Input: part model. Units: mm. Frame: model coordinates. Face numbers are marked on the shaded views. A direction names the side the tool comes from. Give positions to 0.01 mm unless a question says otherwise; leave off trailing zeros. Loops run counter-clockwise (first coordinate to the right, second up) from the corner with the lowest first, then second, coordinate; pieces in that order, holes last. Notation, with made-up numbers: (13, 3) -> (19, 3) arc R25 ccw to (19, 34) -> close; hole circle Ø11 at (-28, 33). An arc over 180 degrees is marked (long way). Answer as a JSON object with one key per item and string values.
Autodesk Fusion 360 part; units mm, degrees
sketch "Sketch1" plane through (0, 0, 0) normal (0, 0, 1) x (1, 0, 0)
  circle A0 centre (0, 0) radius 6.305 construction
  circle A1 centre (0, 0) radius 5.105 construction
  line L0 (0, 0) -> (0, 5.105) construction
  circle A2 centre (0, 5.995) radius 0.89 construction
  circle A3 centre (1.139, 5.9469) radius 0.25 construction
  line L1 (0, 0) -> (2.7356, 5.6806) construction
  line L2 (0, 0) -> (6.305, 0) construction
  circle A4 centre (2.6011, 5.4013) radius 0.89 construction
  circle A5 centre (1.5541, 5.8522) radius 0.25 construction
  arc A6 (0.9079, 5.9375) -> (0.8892, 5.9575) centre (0, 5.105) ccw construction
  arc A7 (0, 5.105) -> (0.8892, 5.9575) centre (0, 5.995) ccw
  arc A8 (1.186, 6.1924) -> (0.8892, 5.9575) centre (1.139, 5.9469) ccw
  arc A9 (1.7837, 5.7533) -> (1.6182, 6.0938) centre (1.5541, 5.8522) ccw
  arc A10 (1.7837, 5.7533) -> (2.215, 4.5994) centre (2.6011, 5.4013) ccw
  line L3 (1.186, 6.1924) -> (1.6182, 6.0938)
  arc A11 (-0.8892, 5.9575) -> (0, 5.105) centre (0, 5.995) ccw
  arc A12 (-0.8892, 5.9575) -> (-1.186, 6.1924) centre (-1.139, 5.9469) ccw
  line L4 (-1.6182, 6.0938) -> (-1.186, 6.1924)
  arc A13 (-1.6182, 6.0938) -> (-1.7837, 5.7533) centre (-1.5541, 5.8522) ccw
  arc A14 (-2.215, 4.5994) -> (-1.7837, 5.7533) centre (-2.6011, 5.4013) ccw
  arc A15 (-3.386, 4.9817) -> (-2.215, 4.5994) centre (-2.6011, 5.4013) ccw
  arc A16 (-3.386, 4.9817) -> (-3.7554, 5.0646) centre (-3.6065, 4.8638) ccw
  line L5 (-4.102, 4.7882) -> (-3.7554, 5.0646)
  arc A17 (-4.102, 4.7882) -> (-4.1033, 4.4096) centre (-3.9393, 4.5983) ccw
  arc A18 (-3.9912, 3.1829) -> (-4.1033, 4.4096) centre (-4.6871, 3.7378) ccw
  arc A19 (-5.2121, 3.0192) -> (-3.9912, 3.1829) centre (-4.6871, 3.7378) ccw
  arc A20 (-5.2121, 3.0192) -> (-5.5809, 2.9337) centre (-5.3596, 2.8173) ccw
  line L6 (-5.7733, 2.5342) -> (-5.5809, 2.9337)
  arc A21 (-5.7733, 2.5342) -> (-5.6102, 2.1926) centre (-5.5444, 2.4337) ccw
  arc A22 (-4.977, 1.136) -> (-5.6102, 2.1926) centre (-5.8447, 1.334) ccw
  arc A23 (-6.006, 0.4587) -> (-4.977, 1.136) centre (-5.8447, 1.334) ccw
  arc A24 (-6.006, 0.4587) -> (-6.3011, 0.2217) centre (-6.0513, 0.2129) ccw
  line L7 (-6.3011, -0.2217) -> (-6.3011, 0.2217)
  arc A25 (-6.3011, -0.2217) -> (-6.006, -0.4587) centre (-6.0513, -0.2129) ccw
  arc A26 (-4.977, -1.136) -> (-6.006, -0.4587) centre (-5.8447, -1.334) ccw
  arc A27 (-5.6102, -2.1926) -> (-4.977, -1.136) centre (-5.8447, -1.334) ccw
  arc A28 (-5.6102, -2.1926) -> (-5.7733, -2.5342) centre (-5.5444, -2.4337) ccw
  line L8 (-5.5809, -2.9337) -> (-5.7733, -2.5342)
  arc A29 (-5.5809, -2.9337) -> (-5.2121, -3.0192) centre (-5.3596, -2.8173) ccw
  arc A30 (-3.9912, -3.1829) -> (-5.2121, -3.0192) centre (-4.6871, -3.7378) ccw
  arc A31 (-4.1033, -4.4096) -> (-3.9912, -3.1829) centre (-4.6871, -3.7378) ccw
  arc A32 (-4.1033, -4.4096) -> (-4.102, -4.7882) centre (-3.9393, -4.5983) ccw
  line L9 (-3.7554, -5.0646) -> (-4.102, -4.7882)
  arc A33 (-3.7554, -5.0646) -> (-3.386, -4.9817) centre (-3.6065, -4.8638) ccw
  arc A34 (-2.215, -4.5994) -> (-3.386, -4.9817) centre (-2.6011, -5.4013) ccw
  arc A35 (-1.7837, -5.7533) -> (-2.215, -4.5994) centre (-2.6011, -5.4013) ccw
  arc A36 (-1.7837, -5.7533) -> (-1.6182, -6.0938) centre (-1.5541, -5.8522) ccw
  line L10 (-1.186, -6.1924) -> (-1.6182, -6.0938)
  arc A37 (-1.186, -6.1924) -> (-0.8892, -5.9575) centre (-1.139, -5.9469) ccw
  arc A38 (0, -5.105) -> (-0.8892, -5.9575) centre (0, -5.995) ccw
  arc A39 (0.8892, -5.9575) -> (0, -5.105) centre (0, -5.995) ccw
  arc A40 (0.8892, -5.9575) -> (1.186, -6.1924) centre (1.139, -5.9469) ccw
  line L11 (1.6182, -6.0938) -> (1.186, -6.1924)
  arc A41 (1.6182, -6.0938) -> (1.7837, -5.7533) centre (1.5541, -5.8522) ccw
  arc A42 (2.215, -4.5994) -> (1.7837, -5.7533) centre (2.6011, -5.4013) ccw
  arc A43 (3.386, -4.9817) -> (2.215, -4.5994) centre (2.6011, -5.4013) ccw
  arc A44 (3.386, -4.9817) -> (3.7554, -5.0646) centre (3.6065, -4.8638) ccw
  line L12 (4.102, -4.7882) -> (3.7554, -5.0646)
  arc A45 (4.102, -4.7882) -> (4.1033, -4.4096) centre (3.9393, -4.5983) ccw
  arc A46 (3.9912, -3.1829) -> (4.1033, -4.4096) centre (4.6871, -3.7378) ccw
  arc A47 (5.2121, -3.0192) -> (3.9912, -3.1829) centre (4.6871, -3.7378) ccw
  arc A48 (5.2121, -3.0192) -> (5.5809, -2.9337) centre (5.3596, -2.8173) ccw
  line L13 (5.7733, -2.5342) -> (5.5809, -2.9337)
  arc A49 (5.7733, -2.5342) -> (5.6102, -2.1926) centre (5.5444, -2.4337) ccw
  arc A50 (4.977, -1.136) -> (5.6102, -2.1926) centre (5.8447, -1.334) ccw
  arc A51 (6.006, -0.4587) -> (4.977, -1.136) centre (5.8447, -1.334) ccw
  arc A52 (6.006, -0.4587) -> (6.3011, -0.2217) centre (6.0513, -0.2129) ccw
  line L14 (6.3011, 0.2217) -> (6.3011, -0.2217)
  arc A53 (6.3011, 0.2217) -> (6.006, 0.4587) centre (6.0513, 0.2129) ccw
  arc A54 (4.977, 1.136) -> (6.006, 0.4587) centre (5.8447, 1.334) ccw
  arc A55 (5.6102, 2.1926) -> (4.977, 1.136) centre (5.8447, 1.334) ccw
  arc A56 (5.6102, 2.1926) -> (5.7733, 2.5342) centre (5.5444, 2.4337) ccw
  line L15 (5.5809, 2.9337) -> (5.7733, 2.5342)
  arc A57 (5.5809, 2.9337) -> (5.2121, 3.0192) centre (5.3596, 2.8173) ccw
  arc A58 (3.9912, 3.1829) -> (5.2121, 3.0192) centre (4.6871, 3.7378) ccw
  arc A59 (4.1033, 4.4096) -> (3.9912, 3.1829) centre (4.6871, 3.7378) ccw
  arc A60 (4.1033, 4.4096) -> (4.102, 4.7882) centre (3.9393, 4.5983) ccw
  line L16 (3.7554, 5.0646) -> (4.102, 4.7882)
  arc A61 (3.7554, 5.0646) -> (3.386, 4.9817) centre (3.6065, 4.8638) ccw
  arc A62 (2.215, 4.5994) -> (3.386, 4.9817) centre (2.6011, 5.4013) ccw
  dimension "d1" = 12.61
  dimension "d2" = 10.21
  dimension "d3" = 1.78
  dimension "d4" = 0.5
  dimension "d6" = 25.714
  dimension "d7" = 1.78
  dimension "d8" = 0.5
  dimension "d10" = 360
extrude "Extrude1" add sketch "Sketch1" along normal blind 10
equation "d2 = d1 - ( ( 2 * 1.2 ) * 1 mm )"
equation "d7 = d3"
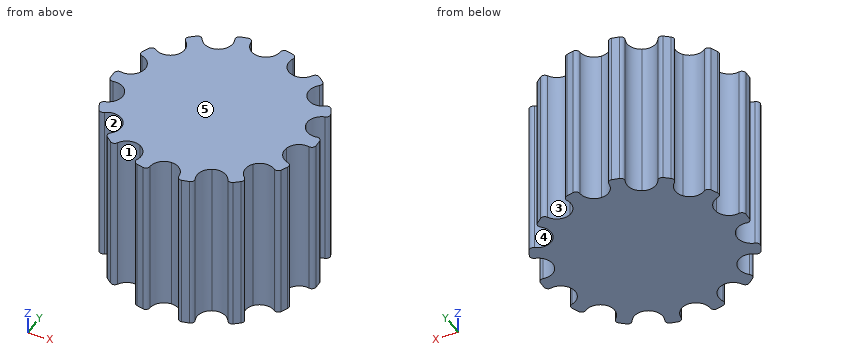
Q1. Section B-B, the plane x = -0.5. Return the cut outline in (y, z), then the cut area to 3 significant figures.
Evaluation:
{"outline": "(-5.26, 0) -> (5.26, 0) -> (5.26, 10) -> (-5.26, 10) -> close", "area": "105 mm2"}
Q2. Draft query along Y for the marked faces 3, 4 and 5. Return one class per face: +Y half, -Y half, draft (parallel to the pull), parting line (faces both ways), or undercut.
Evaluation:
{"face 3": "+Y half", "face 4": "undercut", "face 5": "draft"}
Q3. Ray query, line 1 along Y through (x, z) = (4, 4.5); line 2 along Y through (x, z) = (-3.75, 2.75); line 3 along X through (y, z) = (0.25, 9.25). Return the intervals inside material, ascending.
Evaluation:
{"line 1": "y = -4.87 to -4.3, -3.17 to 3.17, 4.3 to 4.87", "line 2": "y = -5.07 to 5.07", "line 3": "x = -6.3 to 6.3"}
Q4. Section A-A, the plane y = 4. Return the cut outline in (x, z).
Evaluation:
{"outline": "(-3.84, 0) -> (3.84, 0) -> (3.84, 10) -> (-3.84, 10) -> close"}
Q5. Access query for the marked faces 1 and 2. Directions: +Z, -Z, +X, -X, +Y, -Y. A direction counts if a zero-diameter tool reaches every point of the face in a straight line with its end or side. Return the directions, or none.
Evaluation:
{"face 1": "+Z, -Z, -Y", "face 2": "+Z, -Z"}
Q6. Pin query (flat end, axial travel): pin 1 (6 mm diameter, centred on y = 4.5, z = 3.5, fed in from +X). Return the tip coordinate at first contact, or that it passes through.
Evaluation:
{"pin 1": "stops at x = 5.79"}
